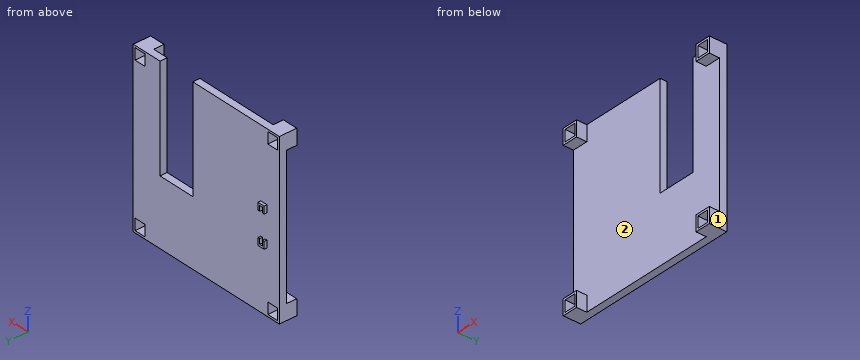
Autodesk Inventor part; units mm, degrees
ref_plane "YZ Plane" through (0, 0, 0) normal (1, 0, 0) x (0, 1, 0)
ref_plane "XZ Plane" through (0, 0, 0) normal (0, 1, 0) x (-1, 0, 0)
ref_plane "XY Plane" through (0, 0, 0) normal (0, 0, 1) x (1, 0, 0)
sketch "Sketch1" plane through (0, 0, 0) normal (0, 1, 0) x (-1, 0, 0)
  line L0 (0, 0) -> (-165, 0)
  line L1 (-165, 0) -> (-165, 165)
  line L2 (-165, 165) -> (0, 165)
  line L3 (0, 165) -> (0, 0)
  line L4 (-165, 165) -> (-150, 165)
  line L5 (-165, 150) -> (-165, 165)
  line L6 (-163, 152) -> (-152, 152)
  line L7 (-152, 152) -> (-152, 163)
  line L8 (-152, 163) -> (-163, 163)
  line L9 (-163, 163) -> (-163, 152)
  line L10 (-2, 152) -> (-13, 152)
  line L11 (-13, 152) -> (-13, 163)
  line L12 (-13, 163) -> (-2, 163)
  line L13 (-2, 163) -> (-2, 152)
  line L14 (-163, 13) -> (-152, 13)
  line L15 (-152, 13) -> (-152, 2)
  line L16 (-152, 2) -> (-163, 2)
  line L17 (-163, 2) -> (-163, 13)
  line L18 (-2, 13) -> (-13, 13)
  line L19 (-13, 13) -> (-13, 2)
  line L20 (-13, 2) -> (-2, 2)
  line L21 (-2, 2) -> (-2, 13)
  line L22 (-150, 150) -> (-165, 150)
  line L23 (-165, 150) -> (-165, 165)
  line L24 (-165, 165) -> (-150, 165)
  line L25 (-150, 165) -> (-150, 150)
  line L26 (-150, 15) -> (-165, 15)
  line L27 (-165, 15) -> (-165, 0)
  line L28 (-165, 0) -> (-150, 0)
  line L29 (-150, 0) -> (-150, 15)
  line L30 (-15, 15) -> (0, 15)
  line L31 (0, 15) -> (0, 0)
  line L32 (0, 0) -> (-15, 0)
  line L33 (-15, 0) -> (-15, 15)
  line L34 (-15, 150) -> (0, 150)
  line L35 (0, 150) -> (0, 165)
  line L36 (0, 165) -> (-15, 165)
  line L37 (-15, 165) -> (-15, 150)
  line L38 (-165, 165) -> (-133.75, 165)
  line L39 (-133.75, 165) -> (-97.75, 165)
  line L40 (-97.75, 165) -> (-97.75, 64)
  line L41 (-97.75, 64) -> (-133.75, 64)
  line L42 (-133.75, 64) -> (-133.75, 165)
  point P0 (0, 15)
  dimension "d0" = 165
  dimension "d1" = 165
  dimension "d5" = 2
  dimension "d6" = 2
  dimension "d7" = 2
  dimension "d8" = 2
  dimension "d9" = 31.25
  dimension "d10" = 36
  dimension "d11" = 101
extrude "Extrusion1" add sketch "Sketch1" along normal blind 7 contours L0 L29 L26 L1 L22 L25 L2 L42 L41 L40 L37 L34 L3 L30 L33
sketch "Sketch2" plane through (0, 7, 0) normal (0, 1, 0) x (1, 0, 0)
  line L0 (15, -15) -> (0, -15)
  line L1 (15, -15) -> (0, -15)
  line L2 (0, -15) -> (0, 0)
  line L3 (0, 0) -> (15, 0)
  line L4 (15, 0) -> (15, -15)
  line L5 (150, -15) -> (150, 0)
  line L6 (150, -15) -> (165, -15)
  line L7 (165, -15) -> (165, 0)
  line L8 (165, 0) -> (150, 0)
  line L9 (150, 0) -> (150, -15)
  line L10 (150, -150) -> (165, -150)
  line L11 (150, -150) -> (165, -150)
  line L12 (165, -150) -> (165, -165)
  line L13 (165, -165) -> (150, -165)
  line L14 (150, -165) -> (150, -150)
  line L15 (15, -150) -> (0, -150)
  line L16 (0, -150) -> (0, -165)
  line L17 (0, -165) -> (15, -165)
  line L18 (15, -165) -> (15, -150)
  line L19 (2, -163) -> (2, -152)
  line L20 (2, -152) -> (13, -152)
  line L21 (13, -152) -> (13, -163)
  line L22 (13, -163) -> (2, -163)
  line L23 (2, -2) -> (2, -13)
  line L24 (2, -13) -> (13, -13)
  line L25 (13, -13) -> (13, -2)
  line L26 (13, -2) -> (2, -2)
  line L27 (163, -2) -> (163, -13)
  line L28 (163, -13) -> (152, -13)
  line L29 (152, -13) -> (152, -2)
  line L30 (152, -2) -> (163, -2)
  line L31 (163, -163) -> (163, -152)
  line L32 (163, -152) -> (152, -152)
  line L33 (152, -152) -> (152, -163)
  line L34 (152, -163) -> (163, -163)
  dimension "d14" = 15
  dimension "d15" = 15
  dimension "d16" = 15
  dimension "d17" = 15
  dimension "d18" = 15
  dimension "d19" = 15
  dimension "d20" = 15
  dimension "d21" = 15
  dimension "d22" = 2
  dimension "d23" = 2
  dimension "d24" = 2
  dimension "d25" = 2
extrude "Extrusion2" add sketch "Sketch2" against normal blind 17
sketch "Sketch3" plane through (0, 7, 0) normal (0, 1, 0) x (1, 0, 0)
  point P0 (0, 0)
surface extrude "ExtrusionSrf1" sketch "Sketch2" against normal blind 37 shown yes curves L21 L22 L19 L20
surface extrude "ExtrusionSrf2" sketch "Sketch2" against normal blind 37 shown yes curves L27 L28 L29 L30
surface extrude "ExtrusionSrf3" sketch "Sketch2" against normal blind 37 shown yes curves L25 L26 L23 L24
surface extrude "ExtrusionSrf4" sketch "Sketch2" against normal blind 37 shown yes curves L31 L32 L33 L34
sketch "Sketch4" plane through (133.75, 0, 64) normal (-1, 0, 0) x (0, 0, 1)
  line L0 (0, 7) -> (101, 7)
  line L1 (101, 0) -> (101, 7)
  line L2 (0, 7) -> (101, 7)
  line L3 (101, 7) -> (101, 0)
  line L4 (101, 0) -> (0, 0)
  line L5 (0, 0) -> (0, 7)
  line L6 (0, 0) -> (0, 7)
  line L7 (0, 7) -> (101, 7)
  line L8 (101, 7) -> (101, 0)
  line L9 (101, 0) -> (0, 0)
  line L10 (0, 0) -> (0, 7)
  point P0 (-64, 0)
extrude "Extrusion3" cut sketch "Sketch4" against normal blind 1
sketch "Sketch5" plane through (0, 7, 0) normal (0, 1, 0) x (1, 0, 0)
  line L0 (13, -2) -> (13, -13)
  line L1 (0, 0) -> (0, -165)
  line L2 (16, -67) -> (19, -67)
  line L3 (19, -67) -> (19, -62)
  line L4 (19, -62) -> (16, -62)
  line L5 (16, -62) -> (16, -67)
  line L6 (21, -60) -> (21, -67)
  line L7 (14, -67) -> (14, -60)
  line L8 (14, -60) -> (21, -60)
  line L9 (21, -67) -> (14, -67)
  line L10 (19, -90.9991) -> (19, -95.9991)
  line L11 (19, -95.9991) -> (16, -95.9991)
  line L12 (16, -95.9991) -> (16, -90.9995)
  line L13 (21, -97.9995) -> (21, -90.9991)
  line L14 (14, -90.9995) -> (14, -97.9995)
  line L15 (14, -97.9995) -> (21, -97.9995)
  line L16 (19, -90.9991) -> (19, -95.9991)
  line L17 (16, -95.9991) -> (16, -90.9995)
  line L18 (14, -90.9995) -> (14, -97.9995)
  line L19 (21, -97.9995) -> (21, -90.9991)
  line L20 (19, -67) -> (21, -67)
  line L21 (21, -60) -> (14, -60)
  line L22 (14, -67) -> (16, -67)
  line L23 (16, -62) -> (19, -62)
  line L24 (19, -90.9991) -> (21, -90.9991)
  line L25 (16, -90.9995) -> (14, -90.9995)
  line L26 (14, -97.9995) -> (16, -97.9995)
  line L27 (16, -97.9995) -> (16, -90.9995)
  line L28 (16, -90.9995) -> (14, -90.9995)
  line L29 (14, -90.9995) -> (14, -97.9995)
  line L30 (16, -97.9995) -> (21, -97.9995)
  line L31 (21, -97.9995) -> (21, -95.9991)
  line L32 (21, -95.9991) -> (16, -95.9991)
  line L33 (16, -95.9991) -> (16, -97.9995)
  line L34 (21, -90.9991) -> (19, -90.9991)
  line L35 (19, -90.9991) -> (19, -95.9991)
  line L36 (19, -95.9991) -> (21, -95.9991)
  line L37 (21, -95.9991) -> (21, -90.9991)
  line L38 (19, -67) -> (21, -67)
  line L39 (21, -67) -> (21, -60)
  line L40 (21, -60) -> (19, -60)
  line L41 (19, -60) -> (19, -67)
  line L42 (19, -60) -> (14, -60)
  line L43 (14, -60) -> (14, -62)
  line L44 (14, -62) -> (19, -62)
  line L45 (19, -62) -> (19, -60)
  line L46 (16, -62) -> (14, -62)
  line L47 (14, -62) -> (14, -67)
  line L48 (14, -67) -> (16, -67)
  line L49 (16, -67) -> (16, -62)
  dimension "d42" = 3
  dimension "d43" = 5
  dimension "d44" = 2
extrude "Extrusion4" add sketch "Sketch5" along normal blind 2.7 contours L9 L7 L44 L5 | L3 L41 L8 L6 L9 | L44 L7 L8 L41 L4 | L24 L13 L32 L10 | L32 L13 L15 L27 L11 | L27 L15 L14 L25 L12
properties part number "piano superiore"
Geometry check sheet. Reference: the model listing, model coordinates, mm. Face numbers are marked on the shaded views. Coordinates: 2 decimals unless noted, no trailing zeros. Order: outer loops, then holes, each group sorted by start corner. A loop starts at its lowest first (then second) coordinate and runs counter-clockwise, first axis right, second up. Notation, with made-up numbers: M -6.5,16.5 L 27.5,16.5 A28 ccw 27.5,35.5 Z; hole C 43,64 d2. An arc over 180 degrees is marked long. One line per question, with ' | ' between items. Start each with the question number.
Item 1: Cross-section at B-B on x = 154.5. Enter the section's corners in (y, z).
Item 2: Cross-section at A-A on y = 5. Enter the section's corners in (x, z), then the cut area to 3 significant figures.
Item 3: Draft check along Z on the marked faces 1 and 2. Enter one of: pulls with the +Z half, pulls with the -Z half, needs draft (parallel to the pull), parting line crosses it, or undercut.
Item 4: Cross-section at C-C on z = 147. Enter the section's corners in (x, y), then the cut area to 3 significant figures.
Item 5: Material ranges on L1, parallel to X at y = 6, z = 107.5; L2, parallel to Y at x = 125, z = 41; L3, parallel to Z at x = 123, y = 6, recorded low to high. Write a range as [from, to].
Item 6: Cross-section at D-D on z = 43.5. Enter the section's corners in (x, y).
Item 7: Gauge pin test, flat ends, axial feed: pin 1 (2 mm diameter, centred on x = 18.5, y = 8.5, fed in from +Z); pin 2 (0.8 mm diameter, centred on y = 8, z = 94, fed in from -X); pin 3 (3.5 mm diameter, centred on y = 2.5, z = 129.5, fed in from -X); pin 4 (1.3 mm diameter, centred on x = 17, y = 8, fed in from -Z). Record the tip position at first contact, or that the pin passes through.
Findings:
1) outline: M -10,0 L 7,0 L 7,2 L -10,2 Z; M -10,13 L 7,13 L 7,152 L -10,152 L -10,150 L 0,150 L 0,15 L -10,15 Z; M -10,163 L 7,163 L 7,165 L -10,165 Z
2) outline: M 0,0 L 165,0 L 165,165 L 134.75,165 L 134.75,64 L 97.75,64 L 97.75,165 L 0,165 Z; hole M 2,2 L 13,2 L 13,13 L 2,13 Z; hole M 2,152 L 13,152 L 13,163 L 2,163 Z; hole M 152,2 L 163,2 L 163,13 L 152,13 Z; hole M 152,152 L 163,152 L 163,163 L 152,163 Z | area: 23,000 mm²
3) face 1: needs draft | face 2: undercut
4) outline: M 0,0 L 97.75,0 L 97.75,7 L 0,7 Z; M 134.75,0 L 165,0 L 165,7 L 134.75,7 Z | area: 896 mm²
5) L1: x = [0, 97.75], [134.75, 165] | L2: y = [0, 7] | L3: z = [0, 64]
6) outline: M 0,0 L 165,0 L 165,7 L 0,7 Z
7) pin 1: stops at z = 98 | pin 2: stops at x = 14 | pin 3: stops at x = 0 | pin 4: stops at z = 60
